Can you work these out from the drawing? Everything is in mm from the part's minimum corner. Give positions to 0.01 mm unless a question says otherwise; leave off trailing zeros. Order: outer loops, then holes, each group sorted by start corner. A loop starts at its lowest first (then second) coordinate and runs counter-clockwise, first axis right, second up. Notation, with made-up numbers: M -10,21.25 L -2,21.25 A30 cw -2,59.25 Z; hole C 40.5,-33 d4. An arc over 180 degrees is marked long. Use a Markdown table: item, result. Add a question column.
Item 1: If I drill on L1, parallel to Y at x = 9.25, z = 4.5; L2, parallel to Y at x = 9.75, z = 6.25; L3, parallel to X at y = 41, z = 2, over which ranges is the centre line in solid material (lowest first)? Write a range as from..to.
Item 2: Suppose I cut it at A-A on y = 27. Write out the boundary of the cut face in (x, z).
Item 3: I'm going to push flat-ended pins straight in: pin 1 Ø2 at (x, y) = (7, 8.5) entering from -Z; pin 2 Ø3 at (x, y) = (2, 34) entering from +Z; pin 3 Ø1 at (y, z) = (29, 6) entering from +X. Where does each tip first touch, or does it pass through?
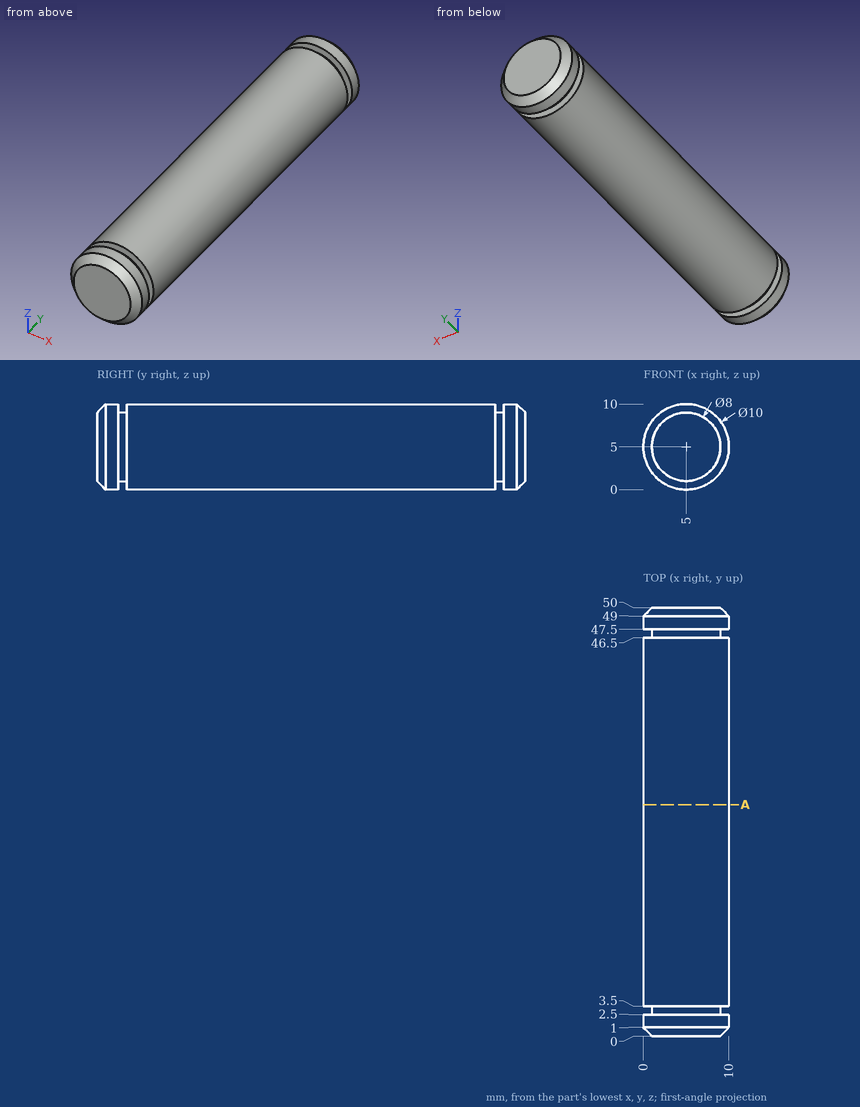
Findings below:
| question | item | result |
|---|---|---|
| 1 | L1 | y = 0.28..2.5, 3.5..46.5, 47.5..49.72 |
| 1 | L2 | y = 0.91..2.5, 3.5..46.5, 47.5..49.09 |
| 1 | L3 | x = 1..9 |
| 2 | outline | C 5,5 d10 |
| 3 | pin 1 | stops at z = 0.1 |
| 3 | pin 2 | stops at z = 9.77 |
| 3 | pin 3 | stops at x = 9.97 |
